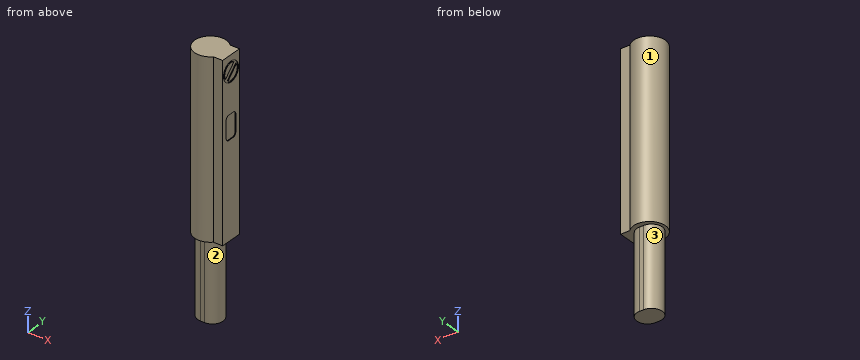
from build123d import *

# Parameters (mm, degrees)
EXTRUDE_1_DEPTH     = 22
EXTRUDE_2_DEPTH     = 10
SKETCH_3_R          = 1.25
SKETCH_3_R_2        = 1.05
CUT_EXTRUDE_1_DEPTH = 0.1
CUT_EXTRUDE_2_DEPTH = 0.1
CUT_EXTRUDE_3_DEPTH = 0.1


with BuildPart() as part:
    # 草图1 → 凸台-拉伸1 (new body)
    with BuildSketch(Plane.XY):
        with BuildLine():
            Line((1.428285686, -1.4), (2.6, -1.4))
            Line((2.6, -1.4), (2.6, 1.4))
            Line((2.6, 1.4), (1.428285686, 1.4))
            ThreePointArc((1.428285686, 1.4), (-2, 0), (1.428285686, -1.4))
        make_face()
    extrude(amount=-EXTRUDE_1_DEPTH)

    # 草图2 → 凸台-拉伸2 (add)
    with BuildSketch(Plane.XY.offset(-22)):
        with BuildLine():
            Line((-0.25, -1.35), (0.25, -1.35))
            ThreePointArc((0.25, -1.35), (1.6, 0), (0.25, 1.35))
            Line((0.25, 1.35), (-0.25, 1.35))
            ThreePointArc((-0.25, 1.35), (-1.6, 0), (-0.25, -1.35))
        make_face()
    extrude(amount=-EXTRUDE_2_DEPTH)

    # 草图3 → 切除-拉伸1 (cut)
    with BuildSketch(Plane(origin=(2.6, 0, 0), x_dir=(0, 0, -1), z_dir=(1, 0, 0))):
        with Locations((2, 0)):
            Circle(SKETCH_3_R)
        with Locations((2, 0)):
            Circle(SKETCH_3_R_2, mode=Mode.SUBTRACT)
    extrude(amount=-CUT_EXTRUDE_1_DEPTH, mode=Mode.SUBTRACT)

    # 草图4 → 切除-拉伸2 (cut)
    with BuildSketch(Plane(origin=(2.6, 0, 0), x_dir=(0, 0, -1), z_dir=(1, 0, 0))):
        with BuildLine():
            Line((7.4, -0.8), (9.6, -0.8))
            ThreePointArc((9.6, -0.8), (9.882842712, -0.682842712), (10, -0.4))
            Line((10, -0.4), (10, 0.4))
            ThreePointArc((10, 0.4), (9.882842712, 0.682842712), (9.6, 0.8))
            Line((9.6, 0.8), (7.4, 0.8))
            ThreePointArc((7.4, 0.8), (7.117157288, 0.682842712), (7, 0.4))
            Line((7, 0.4), (7, -0.4))
            ThreePointArc((7, -0.4), (7.117157288, -0.682842712), (7.4, -0.8))
        make_face()
    extrude(amount=-CUT_EXTRUDE_2_DEPTH, mode=Mode.SUBTRACT)

    # 草图5 → 切除-拉伸3 (cut)
    with BuildSketch(Plane(origin=(2.6, 0, 0), x_dir=(0, 0, -1), z_dir=(1, 0, 0))):
        with BuildLine():
            Line((0.966284129, 0.609451802), (2.609451802, -1.033715871))
            ThreePointArc((2.609451802, -1.033715871), (2.848528137, -0.848528137), (3.033715871, -0.609451802))
            Line((3.033715871, -0.609451802), (1.390548198, 1.033715871))
            ThreePointArc((1.390548198, 1.033715871), (1.151471863, 0.848528137), (0.966284129, 0.609451802))
        make_face()
    extrude(amount=-CUT_EXTRUDE_3_DEPTH, mode=Mode.SUBTRACT)


solid = part.part
Work out the finished part from the listing and answer in its coordinate system (mm). Face numbers are marked on the shaded views. A direction names the side the tool comes from. Give positions to 0.01 mm unless a question says otherwise; leave off trailing zeros. Order: outer loops, then holes, each group sorted by start corner. A loop starts at its lowest first (then second) coordinate and runs counter-clockwise, first axis right, second up. Notation, with made-up numbers: (79.5, 40) -> (96.5, 40) arc R20 ccw to (96.5, 62) -> close; hole circle Ø2 at (-1.75, 63.5). An arc over 180 degrees is marked (long way). Answer as a JSON object with one key per item and string values. Group by question number.
1. Section A-A on z = -19 is taken. Determine the outline of the cut face in (x, y), plus the area to 3 significant figures.
2. Section B-B on x = 2.05 is taken. Determine the outline of the cut face in (y, z), plus the area to 3 significant figures.
3. Section C-C on y = 0 is taken. Determine the outline of the cut face in (x, z), plus the area to 3 significant figures.
4. A tool of negligible diameter and unlimited length cuts with its end or side. For the marked faces 1, 2 and 3, from which of +Z, -Z, +X, -X, +Y, -Y can it reach the whole face along a straight path? Write none if from no direction.
5. Flat-ended cylindrical pins translate along their axes: pin 1 Ø1 at (y, z) = (0, -25) entering from -X; pin 2 Ø2 at (x, z) = (1, -15) entering from +Y; pin 3 Ø0.9 at (x, z) = (2, -5.5) entering from -Y; pin 4 Ø1.3 at (x, z) = (2, -12.5) entering from +Y. Find the tip coordinate at first contact, or state that the pin passes through.
6. Consider line 1 along Y through (x, z) = (2.55, -2); line 2 along X through (y, z) = (0.15, -8.5); line 3 along Z through (x, y) = (-0.25, 1.5). Determine where each line is inside the solid, lowest interval first. Write a range as [from, to].
Result sheet:
{
 "1": {"outline": "(1.43, -1.4) -> (2.6, -1.4) -> (2.6, 1.4) -> (1.43, 1.4) arc R2 ccw (long way) to start", "area": "14.7 mm^2"},
 "2": {"outline": "(-1.4, -22) -> (1.4, -22) -> (1.4, 0) -> (-1.4, 0) -> close", "area": "61.6 mm^2"},
 "3": {"outline": "(-2, -22) -> (-1.6, -22) -> (-1.6, -32) -> (1.6, -32) -> (1.6, -22) -> (2.6, -22) -> (2.6, -10) -> (2.5, -10) -> (2.5, -7) -> (2.6, -7) -> (2.6, -3.25) -> (2.5, -3.25) -> (2.5, -3.05) -> (2.6, -3.05) -> (2.6, -2.42) -> (2.5, -2.42) -> (2.5, -1.58) -> (2.6, -1.58) -> (2.6, -0.95) -> (2.5, -0.95) -> (2.5, -0.75) -> (2.6, -0.75) -> (2.6, 0) -> (-2, 0) -> close", "area": "133 mm^2"},
 "4": {"face 1": "+Z, -Z", "face 2": "-Z, +X", "face 3": "-Z, -X"},
 "5": {"pin 1": "stops at x = -1.6", "pin 2": "stops at y = 2", "pin 3": "stops at y = -1.4", "pin 4": "stops at y = 1.48"},
 "6": {"line 1": "y = [-1.4, -1.25], [-1.05, -0.42], [0.42, 1.05], [1.25, 1.4]", "line 2": "x = [-1.99, 2.5]", "line 3": "z = [-22, 0]"}
}
